Autodesk Inventor part; units mm, degrees
ref_plane "YZ Plane" through (0, 0, 0) normal (1, 0, 0) x (0, 1, 0)
ref_plane "XZ Plane" through (0, 0, 0) normal (0, 1, 0) x (-1, 0, 0)
ref_plane "XY Plane" through (0, 0, 0) normal (0, 0, 1) x (1, 0, 0)
ref_plane "Work Plane13" through (0, 3, 0) normal (0, 1, 0) x (1, 0, 0)
sketch "Sketch45" plane through (0, 3, 0) normal (0, 1, 0) x (1, 0, 0)
  line L0 (35, -20) -> (-3, -20)
  line L1 (-3, -20) -> (-3, 20)
  line L2 (-3, 20) -> (35, 20)
  line L3 (35, 20) -> (35, -20)
  point P0 (0, 0)
  dimension "d142" = 38
  dimension "d143" = 40
extrude "Extrusion34" add sketch "Sketch45" along normal blind 30
sketch "Sketch46" plane through (0, 33, 0) normal (0, 1, 0) x (1, 0, 0)
  point P0 (0, 0)
ref_plane "Work Plane11" through (0, 0, 0) normal (0, -1, 0) x (1, 0, 0)
sketch "Sketch47" plane through (0, 0, 0) normal (0, -1, 0) x (1, 0, 0)
  circle A0 centre (16, 0) radius 18
  point P0 (0, 0)
  dimension "d146" = 36
extrude "Extrusion35" cut sketch "Sketch47" against normal blind 30 draft -15
sketch "Sketch48" plane through (0, 33, 0) normal (0, 1, 0) x (1, 0, 0)
  point P0 (0, 0)
sketch "Sketch49" plane through (0, 33, 0) normal (0, 1, 0) x (1, 0, 0)
  circle A0 centre (20, 0) radius 1.1
  point P0 (0, 0)
  dimension "d149" = 2.2
extrude "Extrusion36" cut sketch "Sketch49" against normal through all
ref_plane "Work Plane7" through (35, 3, -20) normal (0, 0, -1) x (-1, 0, 0)
sketch "Sketch58" plane through (35, 3, -20) normal (0, 0, -1) x (-1, 0, 0)
  line L0 (7, 20) -> (27, 20)
  line L1 (27, 20) -> (27, 5)
  line L2 (27, 5) -> (7, 5)
  line L3 (7, 5) -> (7, 20)
  point P0 (35, -3)
  dimension "d156" = 20
  dimension "d157" = 15
extrude "Extrusion38" cut sketch "Sketch58" against normal blind 15
ref_plane "Work Plane4" through (-3, 3, -20) normal (-1, 0, 0) x (0, 0, 1)
sketch "Sketch59" plane through (-3, 3, -20) normal (-1, 0, 0) x (0, 0, 1)
  line L0 (4, 25) -> (8, 25)
  line L1 (8, 25) -> (8, 5)
  line L2 (8, 5) -> (4, 5)
  line L3 (4, 5) -> (4, 25)
  point P0 (20, -3)
  dimension "d160" = 4
  dimension "d161" = 20
extrude "Extrusion39" cut sketch "Sketch59" against normal blind 35
ref_plane "Work Plane1" through (0, 3, 0) normal (0, 1, 0) x (1, 0, 0)
ref_plane "Work Plane6" through (0, 23, 0) normal (0, 1, 0) x (1, 0, 0)
sketch "Sketch62" plane through (-3, 3, -20) normal (-1, 0, 0) x (0, 0, 1)
  circle A0 centre (20, 15) radius 3
  point P0 (20, -3)
  dimension "d172" = 6
extrude "Extrusion42" cut sketch "Sketch62" against normal through all
sketch "Sketch65" plane through (0, 3, 0) normal (0, -1, 0) x (1, 0, 0)
  line L0 (-3, -12) -> (32, -12)
  line L1 (28, -20) -> (28, -16)
  line L2 (3.5815, -12) -> (28, -12)
  line L3 (28, -12) -> (28, -17.2375)
  line L4 (28, -17.2375) -> (3.5815, -17.2375)
  line L5 (3.5815, -17.2375) -> (3.5815, -12)
  point P0 (0, 0)
extrude "Extrusion44" add sketch "Sketch65" against normal blind 5
properties part number "liquid port_only_v05"
The listing builds one solid part. Answer for the finished solid, in the listing's coordinates (mm). A direction names the side the tool comes from. Give positions to 0.01 mm unless a question says otherwise; leave off trailing zeros. Order: outer loops, then holes, each group sorted by start corner. A loop starts at its lowest first (then second) coordinate and runs counter-clockwise, first axis right, second up. Notation, with made-up numbers: (-20.75, 64) - (28.25, 64) arc R23 ccw to (28.25, 83) - close; hole circle Ø6 at (63.25, 11.25). An arc over 180 degrees is marked (long way). One line per item, written item: value. Start each with the question number.
1) The mould has two halves that part along Y. Classify faces 4 (the face through (8, 16, -18)), 5 (the face through (16, 3, -14)), 6 (the face through (18.9, 31.5, 0)): released by +Y, released by -Y, zero draft, split by the parting line, or undercut.
2) Given pin 1 Ø2 at (x, z) = (18, -7) entering from -Y; pin 2 Ø2 at (y, z) = (17, -14.5) entering from -X; pin 3 Ø1.3 at (x, z) = (20, 0) entering from -Y, each flat-ended and moving along its own axis, determine where each tip first touches the part or whether it passes through.
3) Find the intervals of material crossed by L1, parallel to Y at x = 23.5, z = -18; L2, parallel to Z at x = 20, y = 31; L3, parallel to Z at x = -1, y = 18, in increasing order.
4) A cutting plane is placed at D-D on z = 0. Give the vertices of the cut face in (x, y), then the cut area to 3 significant figures.
5) A cutting plane is placed at B-B on y = 18. Give the vertices of the cut face in (x, z).
6) A tool of negligible diameter and unlimited length cuts with its end or side. For faces 1 (the face through (14, 28, -14)), 2 (the face through (28, 17, -9)), 3 (the face through (8, 19, -11)), from which of +Z, -Z, +X, -X, +Y, -Y can it reach the whole face along a straight path? Write none if from no direction.
7) A cutting plane is placed at C-C on x = 16. Give the vertices of the cut face in (y, z).
8) A cutting plane is placed at A-A on z = -13.5. Give the vertices of the cut face in (x, y).
Answer sheet:
1. face 4: undercut
1. face 5: released by -Y
1. face 6: zero draft
2. pin 1: stops at y = 30
2. pin 2: stops at x = 32
2. pin 3: passes through
3. L1: y = 3 to 8, 23 to 33
3. L2: z = -20 to -1.1, 1.1 to 20
3. L3: z = -20 to -16, -12 to -3, 3 to 20
4. outline: (-3, 3) - (-1.2, 3) - (2.02, 15) - (-3, 15) - close; (-3, 21) - (3.63, 21) - (6.04, 30) - (18.9, 30) - (18.9, 33) - (-3, 33) - close; (21.1, 30) - (25.96, 30) - (28.37, 21) - (35, 21) - (35, 33) - (21.1, 33) - close; (29.98, 15) - (33.2, 3) - (35, 3) - (35, 15) - close
4. area: 330 mm2
5. outline: (-3, -20) - (8, -20) - (8, -16) - (-3, -16) - close; (-3, -12) - (8, -12) - (8, -10.47) arc R13.18 cw to (3.17, -3) - (-3, -3) - close; (-3, 3) - (3.17, 3) arc R13.18 cw to (28.83, 3) - (35, 3) - (35, 20) - (-3, 20) - close; (28, -20) - (35, -20) - (35, -3) - (28.83, -3) arc R13.18 cw to (28, -5.44) - (28, -12) - (32, -12) - (32, -16) - (28, -16) - close
6. face 1: -X
6. face 2: -Z
6. face 3: -Z, -Y
7. outline: (3, -20) - (8, -20) - (8, -12) - (3, -12) - close; (3, 17.2) - (30, 9.96) - (30, -9.96) - (23, -11.84) - (23, -12) - (28, -12) - (28, -16) - (23, -16) - (23, -20) - (33, -20) - (33, 20) - (3, 20) - close
8. outline: (-3, 3) - (35, 3) - (35, 33) - (-3, 33) - (-3, 28) - (32, 28) - (32, 8) - (-3, 8) - close
